Geometry: final body of the model. Coordinates: model frame, mm. Face numbers are marked on the shaded views. Give positions to 0.01 mm unless a question says otherwise; leave off trailing zeros. Loops run counter-clockwise (first coordinate to the right, second up) from the corner with the lowest first, then second, coordinate; pieces in that order, holes last. Notation, with made-up numbers: (19.25, -1) -> (76.25, -1) arc R15 ccw to (76.25, 17) -> close; hole circle Ø3 at (37, -27.5). An arc over 180 degrees is marked (long way). One line per question, with ' | ' between items. Start each with the question number.
Item 1: Section A-A on y = 0. Return loops of the section in (x, z), then the cut area to 3 significant figures.
Item 2: Section B-B on x = -3.25. Return loops of the section in (y, z), then the cut area to 3 significant figures.
Item 3: Mould query, pull axis X, two halves, no side actions, for the marked faces 1, 2 and 3. Classes: released by +X, released by -X, zero draft, split by the parting line, or undercut.
Item 4: Pin query (flat end, axial travel): P1, Ø1.5, axis at x = 6.5, z = 12, coming from the +Y side; P2, Ø2, axis at y = 4, z = 27, coming from the -X side; P3, Ø10, axis at x = 7.5, y = 7.5, coming from the +Z side; P4, Ø12, axis at x = -7.5, z = -0.5, coming from the +Y side. Return the tip coordinate at first contact, or that it passes through.
Item 5: Section C-C on z = 51. Return loops of the section in (x, y), then the cut area to 3 significant figures.
Item 6: Material intervals for line 1 along Y through (x, z) = (0, 67.75); line 2 along Z through (x, y) = (1, -6.25); line 3 along Z through (x, y) = (8, -3), sorted ascending. Write a range as [from, to].
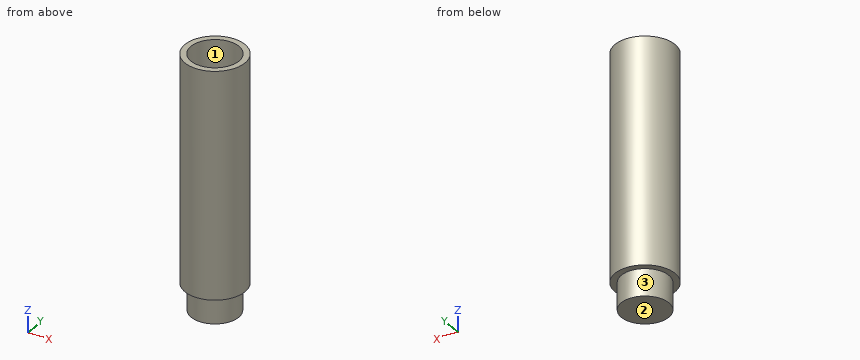
from build123d import *

# Parameters (mm, degrees)
F0_R     = 10
F0_R_2   = 7.9
F1_DEPTH = 75
F2_DEPTH = 9
F3_R     = 8
F4_DEPTH = 10


with BuildPart() as f1:
    # F0 (on Top) → F1 (new body)
    with BuildSketch(Plane.XY):
        Circle(F0_R)
        Circle(F0_R_2, mode=Mode.SUBTRACT)
        Circle(F0_R_2)
    extrude(amount=F1_DEPTH)

    # F0 (on Top) → F2 (join)
    with BuildSketch(Plane.XY):
        Circle(F0_R_2)
    extrude(amount=-F2_DEPTH)

    # F3 (on face) → F4 (cut)
    with BuildSketch(Plane.XY.offset(75)):
        Circle(F3_R)
    extrude(amount=-F4_DEPTH, mode=Mode.SUBTRACT)


solid = f1.part
Result sheet:
1) outline: (-10, 0) -> (-7.9, 0) -> (-7.9, -9) -> (7.9, -9) -> (7.9, 0) -> (10, 0) -> (10, 75) -> (8, 75) -> (8, 65) -> (-8, 65) -> (-8, 75) -> (-10, 75) -> close | area: 1,480 mm²
2) outline: (-9.46, 0) -> (-7.2, 0) -> (-7.2, -9) -> (7.2, -9) -> (7.2, 0) -> (9.46, 0) -> (9.46, 75) -> (7.31, 75) -> (7.31, 65) -> (-7.31, 65) -> (-7.31, 75) -> (-9.46, 75) -> close | area: 1,400 mm²
3) face 1: undercut | face 2: zero draft | face 3: split by the parting line
4) P1: stops at y = 8.18 | P2: stops at x = -9.54 | P3: stops at z = 75 | P4: stops at y = 9.88
5) outline: circle Ø20 at (0, 0) | area: 314 mm²
6) line 1: y = [-10, -8], [8, 10] | line 2: z = [-9, 65] | line 3: z = [0, 75]
